Geometry check sheet. Reference: the model listing, model coordinates, mm. A direction names the side the tool comes from. Give positions to 0.01 mm unless a question says otherwise; leave off trailing zeros. Loops run counter-clockwise (first coordinate to the right, second up) from the corner with the lowest first, then second, coordinate; pieces in that order, holes last. Notation, with made-up numbers: (-31.75, 61) -> (-15.75, 61) arc R19 cw to (-15.75, 84) -> close; hole circle Ø6 at (-3.75, 31.25). An arc over 180 degrees is marked (long way). Write item = value, one per line.
```python
from build123d import *

# Parameters (mm, degrees)
F0_W     = 60
F0_H     = 60
F1_DEPTH = 10
F2_R     = 10
F4_D     = 10
F4_DEPTH = 10
F4_TIP   = 3.0043030951
F5_R     = 16
F6_DEPTH = 20
F8_D     = 17.5
F8_DEPTH = 30
F8_TIP   = 5.2575304165


with BuildPart() as f1:
    # F0 (on Top) → F1 (new body)
    with BuildSketch(Plane.XY):
        Rectangle(F0_W, F0_H)
    extrude(amount=F1_DEPTH)

    # F2
    f2_edges = [f1.edges().sort_by_distance(p)[0] for p in [
        (-30, 30, 5),
        (-30, -30, 5),
        (30, -30, 5),
        (30, 30, 5),
    ]]
    fillet(f2_edges, radius=F2_R)

    # F4
    with Locations(Plane.XY.offset(10)):
        with Locations((-20, 20), (20, 20), (20, -20), (-20, -20)):
            Hole(F4_D / 2, depth=F4_DEPTH)
            with Locations((0, 0, -(F4_DEPTH + F4_TIP / 2))):  # 118° drill point
                Cone(0, F4_D / 2, F4_TIP, mode=Mode.SUBTRACT)

    # F5 (on face) → F6 (join)
    with BuildSketch(Plane.XY.offset(10)):
        Circle(F5_R)
    extrude(amount=F6_DEPTH)

    # F8
    with Locations(Plane.XY.offset(30)):
        with Locations((0, 0)):
            Hole(F8_D / 2, depth=F8_DEPTH)
            with Locations((0, 0, -(F8_DEPTH + F8_TIP / 2))):  # 118° drill point
                Cone(0, F8_D / 2, F8_TIP, mode=Mode.SUBTRACT)


solid = f1.part
```
Item 1: Section check C-C, the plane z = 9.25. Record the cut outline in (x, y), plus the area to 3 significant figures.
Answer:
outline = (-30, -20) arc R10 ccw to (-20, -30) -> (20, -30) arc R10 ccw to (30, -20) -> (30, 20) arc R10 ccw to (20, 30) -> (-20, 30) arc R10 ccw to (-30, 20) -> close; hole circle Ø10 at (-20, -20); hole circle Ø10 at (-20, 20); hole circle Ø17.5 at (0, 0); hole circle Ø10 at (20, -20); hole circle Ø10 at (20, 20)
area = 2,960 mm^2
Item 2: Section check A-A, the plane y = 0. Record the cut outline in (x, z).
Answer:
outline = (-30, 0) -> (-8.75, 0) -> (-8.75, 30) -> (-16, 30) -> (-16, 10) -> (-30, 10) -> close; (8.75, 0) -> (30, 0) -> (30, 10) -> (16, 10) -> (16, 30) -> (8.75, 30) -> close
Item 3: Thickness scan on L1, parallel to X at y = -20, z = 3.75; L2, parallel to Y at x = 0, z = 13. Record the ranges inside material, lowest first. Write a range as [from, to].
Answer:
L1 = [-30, -25], [-15, 15], [25, 30]
L2 = [-16, -8.75], [8.75, 16]
Item 4: Gauge pin test, flat ends, axial feed: pin 1 (8 mm diameter, centred on x = 20, y = -20, fed in from -Z); pin 2 (3 mm diameter, centred on x = -16.5, y = 23, fed in from +Z); pin 3 (1.5 mm diameter, centred on x = 13, z = 26, fed in from +Y); pin 4 (4 mm diameter, centred on y = -9.5, z = 17.5, fed in from -X). Record the tip position at first contact, or that the pin passes through.
Answer:
pin_1 = through
pin_2 = 10
pin_3 = 10.29
pin_4 = -14.13
Item 5: Tool access check on faces 1 (the cylindrical face through (-3.47, -15.62, 19.86)), 2 (the flat face through (0, -30, 5)). Record the directions out of +Z, -Z, +X, -X, +Y, -Y that give a thin tool (end or side, any length) a straight path to the whole face; none if there is none.
Answer:
face_1 = +Z
face_2 = +Z, -Z, +X, -X, -Y
Item 6: Draft check along Y on faces 3 (the cylindrical face through (27.15, 26.99, 5.07)), 4 (the cylindrical face through (26.99, -27.15, 5.07)), 5 (the cylindrical face through (21.08, 15.12, 4.93)). Enter one of: +Y half, -Y half, draft (parallel to the pull), parting line (faces both ways), or undercut.
Answer:
face_3 = +Y half
face_4 = -Y half
face_5 = undercut
Item 7: Section check D-D, the plane y = 18. Record the cut outline in (x, z), plus the area to 3 significant figures.
Answer:
outline = (-30, 0) -> (-24.58, 0) -> (-24.58, 10) -> (-30, 10) -> close; (-15.42, 0) -> (15.42, 0) -> (15.42, 10) -> (-15.42, 10) -> close; (24.58, 0) -> (30, 0) -> (30, 10) -> (24.58, 10) -> close
area = 417 mm^2
